Input: dimensioned drawing with shaded views. Units: mm. Origin: part minimum x, y, z. Coordinates: 2 decimals unless noted, no trailing zeros. Loops run counter-clockwise (first coordinate to the right, second up) from the corner with the lowest first, then second, coordinate; pieces in that order, holes last. Notation, with made-up numbers: (77.25, 31.25) - (132.25, 31.25) arc R20 cw to (132.25, 39.25) - close; hole circle Ø2 at (-7.5, -6). An arc over 180 degrees is marked (long way). Write item = value, one per line. Start each with the question number.
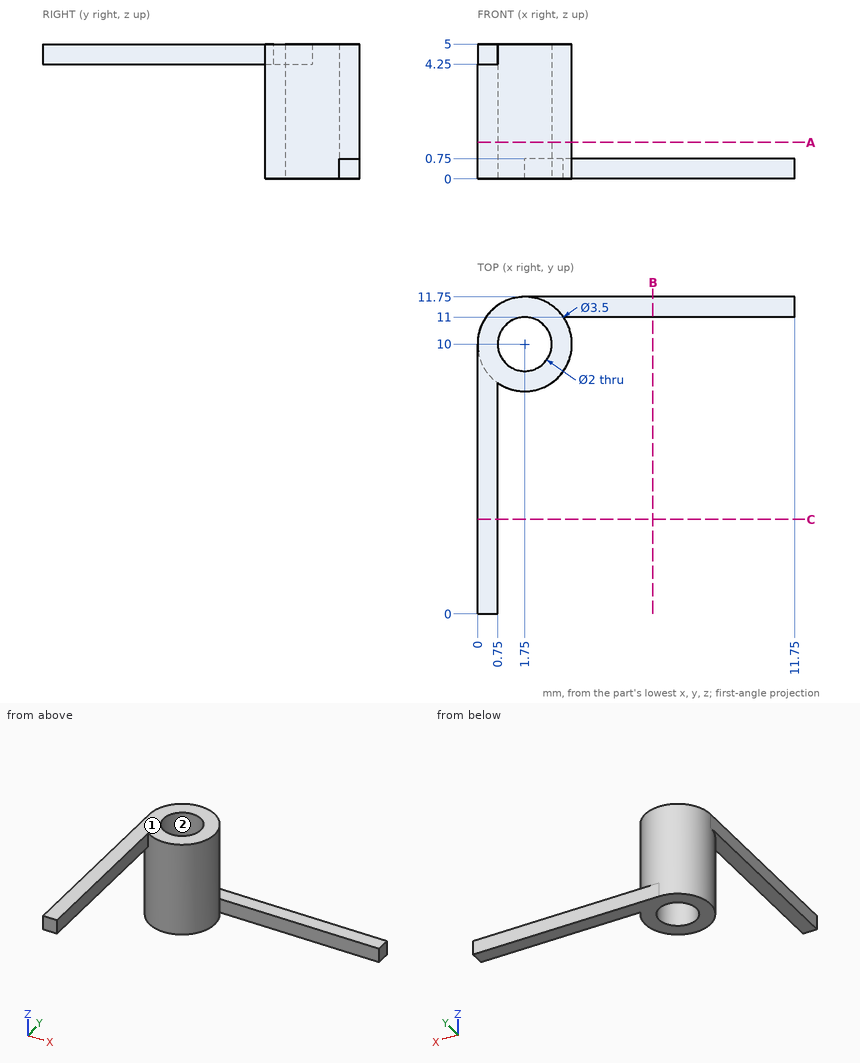
Item 1: Cut plane C-C on y = 3.5. Return loops of the section in (x, z).
Item 2: Cut plane B-B on x = 6.5. Return loops of the section in (y, z).
Item 3: Pull-direction query (Y, two-part tool) for the marked faces 1 and 2; classes: pulls with the +Y half, pulls with the -Y half, needs draft (parallel to the pull), parting line crosses it, or undercut.
Item 4: Cut plane A-A on z = 1.35. Return loops of the section in (x, y), plus the area to 3 significant figures.
Item 5: Pin query (flat end, axial travel): pin 1 (0.8 mm diameter, centred on x = 7.5, y = 11.5, fed in from +Z); pin 2 (0.8 mm diameter, centred on x = 0.5, y = 6.5, fed in from -Z); pin 3 (2 mm diameter, centred on x = 2, y = 6, fed in from -Z); pin 4 (0.6 mm diameter, centred on x = 9, z = 0.5, fed in from -Y). Return the tip coordinate at first contact, or that it passes through.
Item 6: Ray query, line 1 (Y direction, x = 1.75, z = 2.05); line 2 (X direction, y = 10, z = 1.65); line 3 (X direction, y = 10.75, z = 2.6). Return the intervals inside material, ascending.
Recorded:
q1.outline = (0, 4.25) - (0.75, 4.25) - (0.75, 5) - (0, 5) - close
q2.outline = (11, 0) - (11.75, 0) - (11.75, 0.75) - (11, 0.75) - close
q3.face_1 = needs draft
q3.face_2 = undercut
q4.outline = circle Ø3.5 at (1.75, 10); hole circle Ø2 at (1.75, 10)
q4.area = 6.48 mm²
q5.pin_1 = 0.75
q5.pin_2 = 4.25
q5.pin_3 = through
q5.pin_4 = 11
q6.line_1 = 8.25 to 9, 11 to 11.75
q6.line_2 = 0 to 0.75, 2.75 to 3.5
q6.line_3 = 0.17 to 1.09, 2.41 to 3.33
